Verification items for the finished model (mm, model axes). A direction names the side the tool comes from. Give positions to 0.01 mm unless a question says otherwise; leave off trailing zeros. Write each loop counter-clockwise with the first axis right and the second up, starting at its lowest first coordinate (ties: lowest second). Pieces come first, ordered by that corner, then holes. Notation, with made-up numbers: (58, -39.75) -> (68, -39.75) arc R30 ccw to (68, -12.75) -> close; hole circle Ø10 at (82.25, 89). An arc over 180 degrees is marked (long way). Write item = value, one per line.
from build123d import *

# Parameters (mm, degrees)
F0_R             = 13.95
F1_DEPTH         = 46.6
F2_R             = 18.5
F2_R_2           = 13.95
F3_DEPTH         = 24.6
F4_R             = 6
F5_DEPTH         = 6
F6_R             = 3
F7_DEPTH         = 15
F9_DEPTH         = 12
F10_R            = 1.5
F11_DEPTH        = 3.4
F11_COPIES_COUNT = 6


# Not quite as in the source:
# - a pattern or mirror of a feature is missing from the dataset's text; its kind, count and spacing are read off the source's solid


with BuildPart() as f1:
    # F0 (on Front) → F1 (new body)
    with BuildSketch(Plane.XZ):
        Circle(F0_R)
    extrude(amount=F1_DEPTH)

    # F2 (on face) → F3 (join)
    with BuildSketch(Plane.XZ.offset(46.6)):
        Circle(F2_R)
        Circle(F2_R_2, mode=Mode.SUBTRACT)
        Circle(F2_R_2)
    extrude(amount=F3_DEPTH)

    # F4 (on face) → F5 (join)
    with BuildSketch(Plane.XZ.offset(71.2)):
        Circle(F4_R)
    extrude(amount=F5_DEPTH)

    # F6 (on face) → F7 (join)
    with BuildSketch(Plane.XZ.offset(77.2)):
        Circle(F6_R)
    extrude(amount=F7_DEPTH)

    # F8 (on face) → F9 (cut)
    with BuildSketch(Plane.XZ.offset(92.2)):
        with BuildLine():
            Line((-6.2269931659, 8.3767892187), (-6.2269931659, 2.5))
            Line((-6.2269931659, 2.5), (-1.6583123952, 2.5))
            ThreePointArc((-1.6583123952, 2.5), (0, 3), (1.6583123952, 2.5))
            Line((1.6583123952, 2.5), (9.3986019492, 2.5))
            Line((9.3986019492, 2.5), (9.3986019492, 8.3767892187))
            Line((9.3986019492, 8.3767892187), (-6.2269931659, 8.3767892187))
        make_face()
        with BuildLine():
            ThreePointArc((1.6583123952, 2.5), (0, 3), (-1.6583123952, 2.5))
            Line((-1.6583123952, 2.5), (1.6583123952, 2.5))
        make_face()
    extrude(amount=-F9_DEPTH, mode=Mode.SUBTRACT)

    # F10 (on face) → F11 (cut)
    with BuildSketch(Plane.XZ.offset(71.2)):
        with Locations((0, 15.5)):
            Circle(F10_R)
    f11 = extrude(amount=-F11_DEPTH, mode=Mode.SUBTRACT)

    # F11_copies: F11 ×6 about axis
    f11_copies_axis = Axis((0, 0, 0), (0, 1, 0))
    for i in range(1, F11_COPIES_COUNT):
        add(f11.rotate(f11_copies_axis, i * 360 / F11_COPIES_COUNT), mode=Mode.SUBTRACT)


solid = f1.part
Item 1: Sectioned sample at D-D on z = -7.75. Record the cut outline in (x, y).
Response values:
outline = (-16.8, -71.2) -> (-14.92, -71.2) -> (-14.92, -67.8) -> (-11.92, -67.8) -> (-11.92, -71.2) -> (11.92, -71.2) -> (11.92, -67.8) -> (14.92, -67.8) -> (14.92, -71.2) -> (16.8, -71.2) -> (16.8, -46.6) -> (11.6, -46.6) -> (11.6, 0) -> (-11.6, 0) -> (-11.6, -46.6) -> (-16.8, -46.6) -> close
Item 2: Sectioned sample at B-B on y = -82. Record the cut outline in (x, z), then the cut area to 3 significant figures.
Response values:
outline = (-1.66, 2.5) arc R3 ccw (long way) to (1.66, 2.5) -> close
area = 27.1 mm^2
Item 3: Sectioned sample at A-A on z = 0. Record the cut outline in (x, y).
Response values:
outline = (-18.5, -71.2) -> (-6, -71.2) -> (-6, -77.2) -> (-3, -77.2) -> (-3, -92.2) -> (3, -92.2) -> (3, -77.2) -> (6, -77.2) -> (6, -71.2) -> (18.5, -71.2) -> (18.5, -46.6) -> (13.95, -46.6) -> (13.95, 0) -> (-13.95, 0) -> (-13.95, -46.6) -> (-18.5, -46.6) -> close
Item 4: Go/stop test with flat-tipped pins: P1, Ø8, axis at x = 11, z = 14.5, coming from the +Y side; P2, Ø2.5, axis at x = 0, z = -15, coming from the -Y side; P3, Ø0.9, axis at x = 0, z = 16, coming from the -Y side. Record where each tip stops, or that it passes through.
Response values:
P1 = -46.6
P2 = -71.2
P3 = -67.8
Item 5: Material ranges on line 1 (Z direction, x = 0, y = -69.55); line 2 (X direction, y = -69, z = 7); line 3 (Y direction, x = 10.5, z = 13), recorded low to high.
Response values:
line_1 = -18.5 to -17, -14 to 14, 17 to 18.5
line_2 = -17.12 to -14.72, -12.12 to 12.12, 14.72 to 17.12
line_3 = -71.2 to -46.6
Item 6: Sectioned sample at C-C on x = -16. Record the cut outline in (y, z), then the cut area to 3 significant figures.
Response values:
outline = (-71.2, -9.29) -> (-46.6, -9.29) -> (-46.6, 9.29) -> (-71.2, 9.29) -> close
area = 457 mm^2
Item 7: Set-up check for faces 1 (the cylindrical face through (-4.01, -58.73, -18.06)), 2 (the cylindrical face through (1.11, -69.52, -16.51)): record each of +Z, -Z, +X, -X, +Y, -Y from which the full face is reachable in a straight line by a thin tool's end or side.
Response values:
face_1 = +Y, -Y
face_2 = -Y
Item 8: Mould release check, pull along X, two halves, no side actions. Record for faces 3 (the flat face through (0, -92.2, 0)), 4 (the flat face through (0, -67.8, 16)), 5 (the cylindrical face through (-3.02, -22.97, -13.62)): +X half, -X half, draft (parallel to the pull), parting line (faces both ways), or undercut.
Response values:
face_3 = draft
face_4 = undercut
face_5 = parting line
